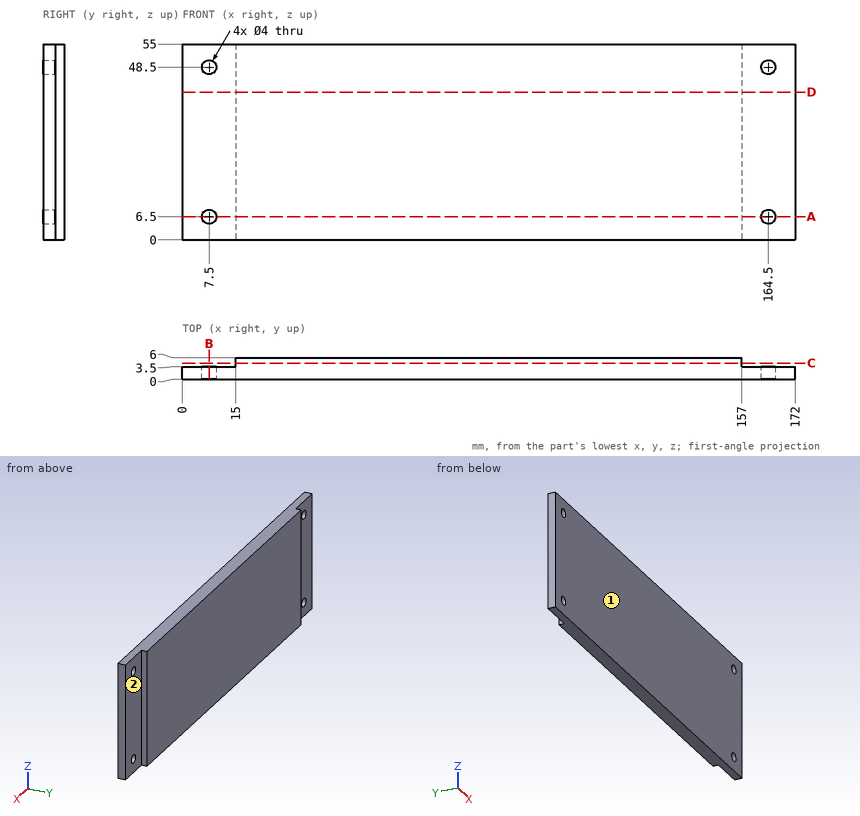
Geometry: see drawing. Coordinates: mm, zero at the bounding-box minimum. A direction names the side the tool comes from. Round coordinates to 2 decimals unless told otherwise and drop trailing zeros. Write each loop counter-clockwise with the first axis right and the second up, starting at its lowest first coordinate (ties: lowest second). Pieces come first, ordered by that corner, then holes. Notation, with made-up numbers: M 24.5,-19 L 33.5,-19 A19 cw 33.5,13 Z; hole C 83.25,-14.75 d3. An arc over 180 degrees is marked long. Answer in a Markdown table with one row per item. Add a question column.
(1) Reachability of the marked faces 1 and 2 from +Z, -Z, +X, -X, +Y, -Y: full face, straight path, thin tool, end or side. Return the list, or none.
(2) Cut plane B-B, the plane x = 7.5. Return the cut outline in (y, z), then the cut area to 4 significant figures.
(3) Contact query for flat-ended pins moving along their axis: pin 1 (0.8 mm diameter, centred on y = 5.5, z = 19, fed in from -X); pin 2 (6.5 mm diameter, centred on x = 7.5, z = 6.5, fed in from +Y). Output: stop coordinate, or through.
(4) Cut plane D-D, the plane z = 41.5. Return the cut outline in (x, y), then the cut area to 3 significant figures.
(5) Cut plane C-C, the plane y = 4.55. Return the cut outline in (x, z), then the cut area to 3 significant figures.
(6) Ray query, L1, parallel to X at y = 0.85, z = 6.5; L2, parallel to Z at x = 7.5, y = 2.55; L3, parallel to X at y = 5, z = 42. Return the intervals inside material, ascending.
(7) Cut plane A-A, the plane z = 6.5. Return the cut outline in (x, y), then the cut area to 3 significant figures.
Established:
| question | item | result |
|---|---|---|
| 1 | face 1 | +Z, -Z, +X, -X, -Y |
| 1 | face 2 | +Z, -Z, +X, +Y |
| 2 | outline | M 0,0 L 3.5,0 L 3.5,4.5 L 0,4.5 Z; M 0,8.5 L 3.5,8.5 L 3.5,46.5 L 0,46.5 Z; M 0,50.5 L 3.5,50.5 L 3.5,55 L 0,55 Z |
| 2 | area | 164.5 mm² |
| 3 | pin 1 | x = 15 |
| 3 | pin 2 | y = 3.5 |
| 4 | outline | M 0,0 L 172,0 L 172,3.5 L 157,3.5 L 157,6 L 15,6 L 15,3.5 L 0,3.5 Z |
| 4 | area | 957 mm² |
| 5 | outline | M 15,0 L 157,0 L 157,55 L 15,55 Z |
| 5 | area | 7,810 mm² |
| 6 | L1 | 0 to 5.5, 9.5 to 162.5, 166.5 to 172 |
| 6 | L2 | 0 to 4.5, 8.5 to 46.5, 50.5 to 55 |
| 6 | L3 | 15 to 157 |
| 7 | outline | M 0,0 L 5.5,0 L 5.5,3.5 L 0,3.5 Z; M 9.5,0 L 162.5,0 L 162.5,3.5 L 157,3.5 L 157,6 L 15,6 L 15,3.5 L 9.5,3.5 Z; M 166.5,0 L 172,0 L 172,3.5 L 166.5,3.5 Z |
| 7 | area | 929 mm² |
